```python
from build123d import *

# Parameters (mm, degrees)
F0_W     = 30
F0_H     = 40
F1_DEPTH = 15
F2_W     = 10
F2_H     = 20
F3_DEPTH = 20
F4_R     = 5
F5_DEPTH = 20.001
F6_R     = 9.99999
F8_DEPTH = 40.001


# Not quite as in the source:
# - a fillet or chamfer is up to 0.001 mm smaller than in the source, because OpenCascade refuses the exact size


with BuildPart() as f1:
    # F0 (on Front) → F1 (new body)
    with BuildSketch(Plane.XZ):
        Rectangle(F0_W, F0_H)
    extrude(amount=F1_DEPTH)

    # F2 (on face) → F3 (join)
    with BuildSketch(Plane.XZ.offset(15)):
        Rectangle(F2_W, F2_H)
    extrude(amount=F3_DEPTH)

    # F4 (on face) → F5 (cut, through all)
    with BuildSketch(Plane.YZ.offset(5)):
        with Locations((-25, 0)):
            Circle(F4_R)
    extrude(amount=-F5_DEPTH, mode=Mode.SUBTRACT)

    # F6 (radius 10 in the source; OpenCascade refuses exactly that, so slightly less here)
    f6_edges = [f1.edges().sort_by_distance(p)[0] for p in [
        (0, -35, 10),
        (0, -35, -10),
    ]]
    fillet(f6_edges, radius=F6_R)

    # F7 (on face) → F8 (cut, through all)
    with BuildSketch(Plane.XY.offset(20)):
        Polygon((15, 0), (-15, 0), (0, -8.6602540378), align=None)
    extrude(amount=-F8_DEPTH, mode=Mode.SUBTRACT)


solid = f1.part
```
The listing builds one solid part. Answer for the finished solid, in the listing's coordinates (mm). A direction names the side the tool comes from. Give positions to 0.01 mm unless a question says otherwise; leave off trailing zeros. Order: outer loops, then holes, each group sorted by start corner. A loop starts at its lowest first (then second) coordinate and runs counter-clockwise, first axis right, second up.
Item 1: The part is cut by section A-A, the plane y = -7. Give the vertices of the cut face in (x, z), and give its area (3 significant figures).
From the geometry:
outline: (-15, -20) - (-2.88, -20) - (-2.88, 20) - (-15, 20) - close; (2.88, -20) - (15, -20) - (15, 20) - (2.88, 20) - close
area: 970 mm2
Item 2: Find the intervals of material crossed by probe 1 along Z at (x, y) = (-2, -25); probe 2 along X at (y, z) = (-8, 2); probe 3 along X at (y, z) = (-28, -9.5), in increasing order.
From the geometry:
probe 1: z = -10 to -5, 5 to 10
probe 2: x = -15 to -1.14, 1.14 to 15
probe 3: x = -5 to 5
Item 3: Given pin 1 Ø5 at (x, y) = (2, -20.5) entering from -Z; pin 2 Ø1.5 at (x, y) = (7.5, -24) entering from +Z (3 decimals); pin 3 Ø12 at (y, z) = (-30, -4.5) entering from +X; pin 4 Ø4 at (x, z) = (3, 7.5) entering from -Y, each flat-ended and moving along its own axis, determine where each tip first touches the part or whether it passes through.
From the geometry:
pin 1: stops at z = -10
pin 2: passes through
pin 3: stops at x = 5
pin 4: stops at y = -33.35
Item 4: The part is cut by section D-D, the plane z = -3. Give the vertices of the cut face in (x, y).
From the geometry:
outline: (-15, -15) - (-5, -15) - (-5, -21) - (5, -21) - (5, -15) - (15, -15) - (15, 0) - (0, -8.66) - (-15, 0) - close; (-5, -34.54) - (5, -34.54) - (5, -29) - (-5, -29) - close
Item 5: The part is cut by section C-C, the plane z = 8. Give the vertices of the cut face in (x, y), and give its area (3 significant figures).
From the geometry:
outline: (-15, -15) - (-5, -15) - (-5, -31) - (5, -31) - (5, -15) - (15, -15) - (15, 0) - (0, -8.66) - (-15, 0) - close
area: 480 mm2
Item 6: Which of the six approach directions +Z, -Z, +X, -X, +Y, -Y give full straight-line access (tool end or side, diameter ignored) to faces 1 (the face through (-5, -20, 2)), 2 (the face through (0, -20, -10)), 3 (the face through (15, -7, 0)), 4 (the face through (-15, -7, 0)), 5 (the face through (0, -20, 10))?
From the geometry:
face 1: +Z, -Z, -X, -Y
face 2: -Z, +X, -X, -Y
face 3: +Z, -Z, +X, +Y, -Y
face 4: +Z, -Z, -X, +Y, -Y
face 5: +Z, +X, -X, -Y
Item 7: For a pull along X with two mould halves and no side action, classify faces 6 (the face through (0.07, -31.99, 7.15)), 7 (the face through (-7.605, -4.27, 0.28)), 8 (the face through (5, -20, 2)), 9 (the face through (7.4, -4.39, 0.28)) as pulls with the +X half, pulls with the -X half, needs draft (parallel to the pull), parting line crosses it, or undercut.
From the geometry:
face 6: needs draft
face 7: undercut
face 8: pulls with the +X half
face 9: undercut
